from build123d import *

# Parameters (mm, degrees)
SKETCH2_R           = 15.875
SKETCH2_R_2         = 2.159
SKETCH2_R_3         = 2.54
BOSS_EXTRUDE1_DEPTH = 3.175
FILLET1_R           = 2.54


with BuildPart() as part:
    # Sketch2 → Boss-Extrude1 (new body)
    with BuildSketch(Plane.XY):
        Polygon((-508, 25.4), (-481.80625, 31.75), (-457.99375, 31.75), (-431.8, 25.4), (-368.3, 25.4), (-368.3, -25.4), (-431.8, -25.4), (-457.99375, -31.75), (-481.80625, -31.75), (-508, -25.4), align=None)
        with Locations((-469.9, 0)):
            Circle(SKETCH2_R, mode=Mode.SUBTRACT)
        with Locations((-457.99375, 20.622229928)):
            Circle(SKETCH2_R_2, mode=Mode.SUBTRACT)
        with Locations((-481.80625, 20.622229928)):
            Circle(SKETCH2_R_2, mode=Mode.SUBTRACT)
        with Locations((-493.7125, 0)):
            Circle(SKETCH2_R_2, mode=Mode.SUBTRACT)
        with Locations((-481.80625, -20.622229928)):
            Circle(SKETCH2_R_2, mode=Mode.SUBTRACT)
        with Locations((-457.99375, -20.622229928)):
            Circle(SKETCH2_R_2, mode=Mode.SUBTRACT)
        with Locations((-446.0875, 0)):
            Circle(SKETCH2_R_2, mode=Mode.SUBTRACT)
        with Locations((-495.3, 12.7)):
            Circle(SKETCH2_R_3, mode=Mode.SUBTRACT)
        with Locations((-495.3, -12.7)):
            Circle(SKETCH2_R_3, mode=Mode.SUBTRACT)
        with Locations((-444.5, -12.7)):
            Circle(SKETCH2_R_3, mode=Mode.SUBTRACT)
        with Locations((-431.8, -12.7)):
            Circle(SKETCH2_R_3, mode=Mode.SUBTRACT)
        with Locations((-419.1, -12.7)):
            Circle(SKETCH2_R_3, mode=Mode.SUBTRACT)
        with Locations((-419.1, 0)):
            Circle(SKETCH2_R_3, mode=Mode.SUBTRACT)
        with Locations((-431.8, 0)):
            Circle(SKETCH2_R_3, mode=Mode.SUBTRACT)
        with Locations((-431.8, 12.7)):
            Circle(SKETCH2_R_3, mode=Mode.SUBTRACT)
        with Locations((-419.1, 12.7)):
            Circle(SKETCH2_R_3, mode=Mode.SUBTRACT)
        with Locations((-444.5, 12.7)):
            Circle(SKETCH2_R_3, mode=Mode.SUBTRACT)
        with Locations((-406.4, 12.7)):
            Circle(SKETCH2_R_3, mode=Mode.SUBTRACT)
        with Locations((-406.4, 0)):
            Circle(SKETCH2_R_3, mode=Mode.SUBTRACT)
        with Locations((-406.4, -12.7)):
            Circle(SKETCH2_R_3, mode=Mode.SUBTRACT)
        with Locations((-393.7, 12.7)):
            Circle(SKETCH2_R_3, mode=Mode.SUBTRACT)
        with Locations((-393.7, 0)):
            Circle(SKETCH2_R_3, mode=Mode.SUBTRACT)
        with Locations((-393.7, -12.7)):
            Circle(SKETCH2_R_3, mode=Mode.SUBTRACT)
        with Locations((-381, 12.7)):
            Circle(SKETCH2_R_3, mode=Mode.SUBTRACT)
        with Locations((-381, 0)):
            Circle(SKETCH2_R_3, mode=Mode.SUBTRACT)
        with Locations((-381, -12.7)):
            Circle(SKETCH2_R_3, mode=Mode.SUBTRACT)
    extrude(amount=BOSS_EXTRUDE1_DEPTH)

    # Fillet1
    fillet1_edges = [part.edges().sort_by_distance(p)[0] for p in [
        (-508, 25.4, 1.5875),
        (-481.80625, 31.75, 1.5875),
        (-457.99375, 31.75, 1.5875),
        (-431.8, 25.4, 1.5875),
        (-368.3, 25.4, 1.5875),
        (-368.3, -25.4, 1.5875),
        (-431.8, -25.4, 1.5875),
        (-457.99375, -31.75, 1.5875),
        (-481.80625, -31.75, 1.5875),
        (-508, -25.4, 1.5875),
    ]]
    fillet(fillet1_edges, radius=FILLET1_R)


solid = part.part
Verification items for the finished model (mm, model axes). A direction names the side the tool comes from. Round coordinates to 2 decimals unless told otherwise and drop trailing zeros. Order: outer loops, then holes, each group sorted by start corner. A loop starts at its lowest first (then second) coordinate and runs counter-clockwise, first axis right, second up. Notation, with made-up numbers: (60.25, 43) -> (76.25, 43) arc R32 ccw to (76.25, 71) -> close; hole circle Ø8 at (-11.5, 31.5). An arc over 180 degrees is marked (long way). Put each result on its own line as item: value.
1) Section check D-D (y = 14). Give the number of separate pieces and of enclosed holes in the cut face, then the cut area to 3 significant figures.
Final values:
separate pieces: 9
enclosed holes: 0
area: 299 mm^2
2) Section check C-C (y = -5). Record the cut outline in (x, z) (3 decimals), then the cut area to 3 significant figures.
Final values:
outline: (-508, 0) -> (-484.967, 0) -> (-484.967, 3.175) -> (-508, 3.175) -> close; (-454.833, 0) -> (-368.3, 0) -> (-368.3, 3.175) -> (-454.833, 3.175) -> close
area: 348 mm^2
3) Material ranges on line 1 (Y direction, x = -393.7, z = 1.35); line 2 (X direction, y = 21, z = 2.2); line 3 (Y direction, x = -385, z = 0.1), recorded low to high.
Final values:
line 1: y = -25.4 to -15.24, -10.16 to -2.54, 2.54 to 10.16, 15.24 to 25.4
line 2: x = -508 to -483.93, -479.68 to -460.12, -455.87 to -368.3
line 3: y = -25.4 to 25.4
4) Section check A-A (x = -469.9). Record the cut outline in (y, z) (3 decimals), then the cut area to 3 significant figures.
Final values:
outline: (-31.75, 0) -> (-15.875, 0) -> (-15.875, 3.175) -> (-31.75, 3.175) -> close; (15.875, 0) -> (31.75, 0) -> (31.75, 3.175) -> (15.875, 3.175) -> close
area: 101 mm^2
5) Set-up check for faces 5 (the flat face through (-401, -25.4, 2)), 6 (the flat face through (-494.248, 28.734, 1.565)), 7 (the flat face through (-402, 25.4, 2)): record each of +Z, -Z, +X, -X, +Y, -Y from which the full face is reachable in a straight line by a thin tool's end or side.
Final values:
face 5: +Z, -Z, +X, -Y
face 6: +Z, -Z, -X, +Y
face 7: +Z, -Z, +X, +Y
6) Section check B-B (x = -406.4). Record the cut outline in (y, z) (3 decimals).
Final values:
outline: (-25.4, 0) -> (-15.24, 0) -> (-15.24, 3.175) -> (-25.4, 3.175) -> close; (-10.16, 0) -> (-2.54, 0) -> (-2.54, 3.175) -> (-10.16, 3.175) -> close; (2.54, 0) -> (10.16, 0) -> (10.16, 3.175) -> (2.54, 3.175) -> close; (15.24, 0) -> (25.4, 0) -> (25.4, 3.175) -> (15.24, 3.175) -> close
7) Mould release check, pull along Y, two halves, no side actions. Record for faces 1 (the flat face through (-437, 0, 0)), 2 (the cylindrical face through (-507.471, -24.954, 1.61)), 3 (the cylindrical face through (-408.938, -12.588, 1.565)), 4 (the cylindrical face through (-378.654, -0.973, 1.565)): +Y half, -Y half, draft (parallel to the pull), parting line (faces both ways), or undercut.
Final values:
face 1: draft
face 2: -Y half
face 3: undercut
face 4: undercut
